Part model, mm, in its own coordinate system. A direction names the side the tool comes from. Round coordinates to 2 decimals unless told otherwise and drop trailing zeros. Write each loop counter-clockwise with the first axis right and the second up, starting at its lowest first coordinate (ties: lowest second). Pieces come first, ordered by that corner, then holes. Notation, with made-up numbers: M 72.5,-4 L 113.5,-4 A17 cw 113.5,11 Z; hole C -17,-26 d7. An arc over 180 degrees is marked long. Answer as a JSON object with one key per item and string values. Group by question number.
1. Band-saw the part on A-A, the plane y = 0. Write the cut outline in (x, z) (3 decimals).
2. Two-plate mould, pull along Z, no slides. Class faces 1 (the face through (-52, 4, -61.468)), 2 (the face through (-27, -53.975, 1)), 3 (the face through (-52, 4, 61.468)), 4 (the face through (-37, -49.975, 34)): +Z half, -Z half, draft (parallel to the pull), parting line (faces both ways), or undercut.
3. Drill centre lines: line 1 (Z direction, x = -38, y = 38); line 2 (Z direction, x = -38, y = -51); line 3 (X direction, y = 1.5, z = 41) (3 decimals). Where is each one in solid material? Low to high. Write a range as from..to.
4. Which spindle directions (+Z, -Z, +X, -X, +Y, -Y) get a long thin tool onto all of the face, cutting with end or side? Do faces 5 (the face through (-53.975, 1, 1)), 6 (the face through (-39.715, 52.003, 28.861)), 7 (the face through (-36.218, -52.003, -29.015)). Say none if no direction does.
5. Band-saw the part on B-B, the plane z = -1. Write the cut outline in (x, y) (3 decimals), plus the area to 3 significant figures.
6. Band-saw the part on D-D, the plane x = 42. Write the cut outline in (y, z), plus the area to 3 significant figures.
7. Drop flat-ended pins along their axis: pin 1 (12 mm diameter, centred on x = 23.5, z = 9.5, fed in from -Y); pin 2 (8 mm diameter, centred on y = 22.5, z = -3.5, fed in from +X); pin 3 (12 mm diameter, centred on y = 6.5, z = -48.5, fed in from +X); pin 4 (7.5 mm diameter, centred on x = -38.5, z = -30.5, fed in from -Y) (3 decimals). Give the stop position or say it passes through.
8. Band-saw the part on C-C, the plane y = -44.5. Write the cut outline in (x, z) (3 decimals).
from build123d import *

# Parameters (mm, degrees)
F0_R     = 50.8
F1_DEPTH = 61.468
F2_R     = 1.7399
F3_DEPTH = 304.8
F4_R     = 3.5
F5_DEPTH = 4
F6_R     = 3.5
F7_DEPTH = 4


with BuildPart() as f1:
    # F0 (on Top) → F1 (new body, symmetric)
    with BuildSketch(Plane.XY):
        with BuildLine():
            Line((-53.975, -53.975), (0, -53.975))
            ThreePointArc((0, -53.975), (53.975, 0), (0, 53.975))
            Line((0, 53.975), (-53.975, 53.975))
            Line((-53.975, 53.975), (-53.975, -53.975))
        make_face()
        Circle(F0_R, mode=Mode.SUBTRACT)
    extrude(amount=F1_DEPTH, both=True)

    # F2 (on face) → F3 (cut)
    with BuildSketch(Plane(origin=(0, 53.975, 0), x_dir=(-1, 0, 0), z_dir=(0, 1, 0))):
        with Locations((38.1, 31.9659)):
            Circle(F2_R)
        with Locations((38.1, -31.9659)):
            Circle(F2_R)
    extrude(amount=-F3_DEPTH, mode=Mode.SUBTRACT)

    # F4 (on face) → F5 (cut)
    with BuildSketch(Plane.XZ.offset(53.975)):
        with Locations((-38.1, 31.9659)):
            Circle(F4_R)
        with Locations((-38.1, -31.9659)):
            Circle(F4_R)
    extrude(amount=-F5_DEPTH, mode=Mode.SUBTRACT)

    # F6 (on face) → F7 (cut)
    with BuildSketch(Plane(origin=(0, 53.975, 0), x_dir=(-1, 0, 0), z_dir=(0, 1, 0))):
        with Locations((38.1, 31.9659)):
            Circle(F6_R)
        with Locations((38.1, -31.9659)):
            Circle(F6_R)
    extrude(amount=-F7_DEPTH, mode=Mode.SUBTRACT)


solid = f1.part
Worked answers:
{
 "1": {"outline": "M -53.975,-61.468 L -50.8,-61.468 L -50.8,61.468 L -53.975,61.468 Z; M 50.8,-61.468 L 53.975,-61.468 L 53.975,61.468 L 50.8,61.468 Z"},
 "2": {"face 1": "-Z half", "face 2": "draft", "face 3": "+Z half", "face 4": "undercut"},
 "3": {"line 1": "z = -61.47..-33.7, -30.23..30.23, 33.7..61.47", "line 2": "z = -61.47..-35.46, -28.47..28.47, 35.46..61.47", "line 3": "x = -53.975..-50.778, 50.778..53.954"},
 "4": {"face 5": "+Z, -Z, -X, +Y, -Y", "face 6": "+Y", "face 7": "-Y"},
 "5": {"outline": "M -53.975,-53.975 L 0,-53.975 A53.975 ccw 0,53.975 L -53.975,53.975 Z; hole C 0,0 d101.6", "area": "2,300 mm^2"},
 "6": {"outline": "M -33.9,-61.47 L -28.58,-61.47 L -28.58,61.47 L -33.9,61.47 Z; M 28.58,-61.47 L 33.9,-61.47 L 33.9,61.47 L 28.58,61.47 Z", "area": "1,310 mm^2"},
 "7": {"pin 1": "stops at y = -51.06", "pin 2": "stops at x = 50.71", "pin 3": "stops at x = 53.97", "pin 4": "stops at y = -53.975"},
 "8": {"outline": "M -53.975,-61.468 L -24.503,-61.468 L -24.503,61.468 L -53.975,61.468 Z; M 24.503,-61.468 L 30.546,-61.468 L 30.546,61.468 L 24.503,61.468 Z; hole C -38.1,-31.966 d3.48; hole C -38.1,31.966 d3.48"}
}
